```python
from build123d import *

# Parameters (mm, degrees)
SKETCH_1_W           = 185
SKETCH_1_H           = 93
SKETCH_1_R           = 1.35
EXTRUDE_1_DEPTH      = 2
SKETCH_2_R           = 2.05
CUT_EXTRUDE_1_DEPTH  = 20
CHAMFER_1_SIZE       = 10
FILLET_1_R           = 1.5
CUT_EXTRUDE_10_DEPTH = 20
CUT_EXTRUDE_11_DEPTH = 20
FILLET_2_R           = 1.5


with BuildPart() as part:
    # 草图1 → 凸台-拉伸1 (new body)
    with BuildSketch(Plane(origin=(0, 0, 0), x_dir=(1, 0, 0), z_dir=(0, 1, 0))):
        Rectangle(SKETCH_1_W, SKETCH_1_H)
        with Locations(Location((-21, 31.5, 0), (0, 0, 270))):
            Circle(SKETCH_1_R, mode=Mode.SUBTRACT)
        with Locations(Location((-21, -31.5, 0), (0, 0, 270))):
            Circle(SKETCH_1_R, mode=Mode.SUBTRACT)
        with Locations(Location((21, -31.5, 0), (0, 0, 270))):
            Circle(SKETCH_1_R, mode=Mode.SUBTRACT)
        with Locations(Location((21, 31.5, 0), (0, 0, 270))):
            Circle(SKETCH_1_R, mode=Mode.SUBTRACT)
    extrude(amount=EXTRUDE_1_DEPTH)

    # 草图2 → 切除-拉伸1 (cut)
    with BuildSketch(Plane(origin=(0, 2, 0), x_dir=(1, 0, 0), z_dir=(0, 1, 0))):
        with Locations(Location((-82.5, 30, 0), (0, 0, 270))):
            Circle(SKETCH_2_R)
        with Locations(Location((82.5, 30, 0), (0, 0, 270))):
            Circle(SKETCH_2_R)
        with Locations(Location((82.5, -30, 0), (0, 0, 270))):
            Circle(SKETCH_2_R)
        with Locations(Location((-82.5, -30, 0), (0, 0, 270))):
            Circle(SKETCH_2_R)
    extrude(amount=-CUT_EXTRUDE_1_DEPTH, mode=Mode.SUBTRACT)

    # 倒角1
    chamfer_1_edges = [part.edges().sort_by_distance(p)[0] for p in [
        (-92.5, 1, -46.5),
        (92.5, 1, -46.5),
        (92.5, 1, 46.5),
        (-92.5, 1, 46.5),
    ]]
    chamfer(chamfer_1_edges, length=CHAMFER_1_SIZE)

    # 圆角1
    fillet_1_edges = [part.edges().sort_by_distance(p)[0] for p in [
        (-82.5, 1, -46.5),
        (82.5, 1, -46.5),
        (92.5, 1, 36.5),
        (92.5, 1, -36.5),
        (-82.5, 1, 46.5),
        (82.5, 1, 46.5),
        (-92.5, 1, -36.5),
        (-92.5, 1, 36.5),
    ]]
    fillet(fillet_1_edges, radius=FILLET_1_R)

    # 草图3 → 切除-拉伸10 (cut)
    with BuildSketch(Plane(origin=(0, 2, 0), x_dir=(1, 0, 0), z_dir=(0, 1, 0))):
        Polygon((-29, 41.5), (-72.5, 41.5), (-29, 25.667294809), align=None)
        Polygon((-29, 21.41058372), (-72.5, 37.24328891), (-72.5, 4.298373792), align=None)
        Polygon((-29, 17.112209927), (-72.5, 0), (-29, -17.112209927), align=None)
        Polygon((-29, -21.41058372), (-72.5, -4.298373792), (-72.5, -37.24328891), align=None)
        Polygon((-29, -25.667294809), (-72.5, -41.5), (-29, -41.5), align=None)
        Polygon((29, -41.5), (72.5, -41.5), (29, -25.667294809), align=None)
        Polygon((29, -21.41058372), (72.5, -37.24328891), (72.5, -4.298373792), align=None)
        Polygon((29, 17.112209927), (29, -17.112209927), (72.5, 0), align=None)
        Polygon((29, 21.41058372), (72.5, 4.298373792), (72.5, 37.24328891), align=None)
        Polygon((29, 41.5), (29, 25.667294809), (72.5, 41.5), align=None)
    extrude(amount=-CUT_EXTRUDE_10_DEPTH, mode=Mode.SUBTRACT)

    # 草图4 → 切除-拉伸11 (cut)
    with BuildSketch(Plane(origin=(0, 2, 0), x_dir=(1, 0, 0), z_dir=(0, 1, 0))):
        Polygon((-13, 41.5), (0, 32.397302003), (13, 41.5), align=None)
        Polygon((0, 27.514203648), (-13, 36.616901645), (-13, 16.616901645), (0, 24.514203648), (13, 16.616901645), (13, 36.616901645), align=None)
        Polygon((-13, 16.616901645), (0, 13.442564884), (13, 16.616901645), (0, 24.514203648), align=None)
        Polygon((0, 10.354424059), (-13, 13.52876082), (-13, 0), (0, 7.354424059), (13, 0), (13, 13.52876082), align=None)
        Polygon((-13, 0), (0, 7.354424059), (13, 0), (0, -7.354424059), align=None)
        Polygon((0, -7.354424059), (-13, 0), (-13, -13.52876082), (0, -10.354424059), (13, -13.52876082), (13, 0), align=None)
        Polygon((0, -13.442564884), (13, -16.616901645), (0, -24.514203648), (-13, -16.616901645), align=None)
        Polygon((0, -24.514203648), (-13, -16.616901645), (-13, -36.616901645), (0, -27.514203648), (13, -36.616901645), (13, -16.616901645), align=None)
        Polygon((0, -32.397302003), (13, -41.5), (-13, -41.5), align=None)
    extrude(amount=-CUT_EXTRUDE_11_DEPTH, mode=Mode.SUBTRACT)

    # 圆角2
    fillet_2_edges = [part.edges().sort_by_distance(p)[0] for p in [
        (-72.5, 1, 37.24328891),
        (-72.5, 1, 4.298373792),
        (-29, 1, 21.41058372),
        (-72.5, 1, 41.5),
        (-29, 1, 25.667294809),
        (-29, 1, 41.5),
        (-29, 1, -21.41058372),
        (-72.5, 1, -4.298373792),
        (-72.5, 1, -37.24328891),
        (-72.5, 1, 0),
        (-29, 1, -17.112209927),
        (-29, 1, 17.112209927),
        (29, 1, -17.112209927),
        (72.5, 1, 0),
        (29, 1, 17.112209927),
        (72.5, 1, -37.24328891),
        (72.5, 1, -4.298373792),
        (29, 1, -21.41058372),
        (72.5, 1, 41.5),
        (29, 1, 41.5),
        (29, 1, 25.667294809),
        (72.5, 1, 4.298373792),
        (72.5, 1, 37.24328891),
        (29, 1, 21.41058372),
        (72.5, 1, -41.5),
        (29, 1, -25.667294809),
        (29, 1, -41.5),
        (-72.5, 1, -41.5),
        (-29, 1, -41.5),
        (-29, 1, -25.667294809),
        (-13, 1, 13.52876082),
        (-13, 1, -13.52876082),
        (0, 1, -10.354424059),
        (13, 1, -13.52876082),
        (13, 1, 13.52876082),
        (0, 1, 10.354424059),
        (-13, 1, -16.616901645),
        (-13, 1, -36.616901645),
        (0, 1, -27.514203648),
        (13, 1, -36.616901645),
        (13, 1, -16.616901645),
        (0, 1, -13.442564884),
        (0, 1, 32.397302003),
        (13, 1, 41.5),
        (-13, 1, 41.5),
        (-13, 1, 16.616901645),
        (0, 1, 13.442564884),
        (13, 1, 16.616901645),
        (13, 1, 36.616901645),
        (0, 1, 27.514203648),
        (-13, 1, 36.616901645),
        (0, 1, -32.397302003),
        (-13, 1, -41.5),
        (13, 1, -41.5),
    ]]
    fillet(fillet_2_edges, radius=FILLET_2_R)


solid = part.part
```
Geometry check sheet. Reference: the model listing, model coordinates, mm. A direction names the side the tool comes from. Coordinates: 2 decimals unless noted, no trailing zeros. Loops run counter-clockwise (first coordinate to the right, second up) from the corner with the lowest first, then second, coordinate; pieces in that order, holes last. Notation, with made-up numbers: (48.5, -39) - (101.5, -39) arc R26 ccw to (101.5, -12) - close; hole circle Ø10 at (66.25, -14). An arc over 180 degrees is marked (long way). One line per item, written item: value. Start each with the question number.
(1) Depth check by flat-ended pin: P1, Ø1, axis at y = 1, z = 37, coming from the +X side. Enter the tip coordinate at first touch or a pass-through.
(2) Cross-section at A-A on x = 57. Enter the section's corners in (y, z).
(3) Material ranges on line 1 (Z direction, x = 30.5, y = 0.35); line 2 (X direction, y = 1.3, z = 0.5); line 3 (X direction, y = 0.2, z = -39), recorded low to high. Write a range as [from, to].
(4) Tool access check on faces 1 (the flat face through (88, 1, 41)), 2 (the flat face through (51.869, 1.014, -29.734)). Record the directions out of +Z, -Z, +X, -X, +Y, -Y that give a thin tool (end or side, any length) a straight path to the whole face; none if there is none.
(5) Cross-section at B-B on y = 1.6. Count the separate pieces of the cut face and the enclosed holes in it, plus the area to 3 significant figures.
(6) Mould release check, pull along X, two halves, no side actions. Record for faces 3 (the flat face through (-87, 1, -42)), 4 (the cylindrical face through (-80.467, 1.014, 29.733)), 5 (the flat face through (-1, 0, -11)): released by +X, released by -X, zero draft, split by the parting line, or undercut.
Results below:
1. P1: stops at x = 92.37
2. outline: (0, -46.5) - (2, -46.5) - (2, -41.5) - (0, -41.5) - close; (0, -35.86) - (2, -35.86) - (2, -31.6) - (0, -31.6) - close; (0, -10.4) - (2, -10.4) - (2, -6.1) - (0, -6.1) - close; (0, 6.1) - (2, 6.1) - (2, 10.4) - (0, 10.4) - close; (0, 31.6) - (2, 31.6) - (2, 35.86) - (0, 35.86) - close; (0, 41.5) - (2, 41.5) - (2, 46.5) - (0, 46.5) - close
3. line 1: z = [-46.5, -41.5], [-26.31, -16.41], [16.41, 26.31], [41.5, 46.5]
3. line 2: x = [-92.5, -69.82], [-29, -13], [13, 29], [69.82, 92.5]
3. line 3: x = [-90, -65.11], [-29, -9.36], [9.36, 29], [65.11, 90]
4. face 1: +Z, +X, +Y, -Y
4. face 2: +Y, -Y
5. separate pieces: 1
5. enclosed holes: 23
5. area: 9,560 mm2
6. face 3: released by -X
6. face 4: undercut
6. face 5: zero draft
